from build123d import *

# Parameters (mm, degrees)
F0_R     = 13.57391
F1_DEPTH = 17
F3_DEPTH = 1.5
F5_DEPTH = 34
F6_R     = 1
F7_R     = 15.57391
F7_R_2   = 13.57391
F8_DEPTH = 1.5
F9_SIZE2 = 0.99999
F9_SIZE  = 1.99999
F10_R    = 1


# Not quite as in the source:
# - a fillet or chamfer is up to 0.001 mm smaller than in the source, because OpenCascade refuses the exact size
# - a feature names something its author has since deleted; it is built from what else it names


with BuildPart() as f1:
    # F0 (on Top) → F1 (new body, symmetric)
    with BuildSketch(Plane.XY):
        Circle(F0_R)
    extrude(amount=F1_DEPTH, both=True)

    # F2 (on Top) → F3 (join, symmetric)
    with BuildSketch(Plane.XY):
        with BuildLine():
            Line((-8.8722387473, 10.27299432), (-13.094084175, 11.721231689))
            ThreePointArc((-13.094084175, 11.721231689), (-13.7398361081, 10.9571536638), (-14.3410637787, 10.1575687241))
            Line((-14.3410637787, 10.1575687241), (-11.9896877566, 6.3638369077))
            ThreePointArc((-11.9896877566, 6.3638369077), (-10.6125101782, 8.4631944563), (-8.8722387473, 10.27299432))
        make_face()
        with BuildLine():
            ThreePointArc((1, 17.5454356654), (0, 17.57391), (-1, 17.5454356654))
            Line((-1, 17.5454356654), (-2.5, 13.3417027657))
            ThreePointArc((-2.5, 13.3417027657), (0, 13.57391), (2.5, 13.3417027657))
            Line((2.5, 13.3417027657), (1, 17.5454356654))
        make_face()
        with BuildLine():
            Line((11.9896877566, 6.3638369077), (14.3410637787, 10.1575687241))
            ThreePointArc((14.3410637787, 10.1575687241), (13.7398361081, 10.9571536638), (13.094084175, 11.721231689))
            Line((13.094084175, 11.721231689), (8.8722387473, 10.27299432))
            ThreePointArc((8.8722387473, 10.27299432), (10.6125101782, 8.4631944563), (11.9896877566, 6.3638369077))
        make_face()
        with BuildLine():
            Line((12.4508960874, -5.4061279404), (16.8830140276, -4.8791546431))
            ThreePointArc((16.8830140276, -4.8791546431), (17.1332953852, -3.9105628665), (17.3280558955, -2.9292988187))
            Line((17.3280558955, -2.9292988187), (13.5635007572, -0.5314883795))
            ThreePointArc((13.5635007572, -0.5314883795), (13.2335837364, -3.0204791306), (12.4508960874, -5.4061279404))
        make_face()
        with BuildLine():
            Line((3.5363257124, -13.1051681845), (6.711710363, -16.2417750474))
            ThreePointArc((6.711710363, -16.2417750474), (7.6250337817, -15.8335457973), (8.5136480988, -15.3740075692))
            Line((8.5136480988, -15.3740075692), (8.0411700519, -10.9357494889))
            ThreePointArc((8.0411700519, -10.9357494889), (5.8894988252, -12.2296703257), (3.5363257124, -13.1051681845))
        make_face()
        with BuildLine():
            Line((-8.0411700519, -10.9357494889), (-8.5136480988, -15.3740075692))
            ThreePointArc((-8.5136480988, -15.3740075692), (-7.6250337817, -15.8335457973), (-6.711710363, -16.2417750474))
            Line((-6.711710363, -16.2417750474), (-3.5363257124, -13.1051681845))
            ThreePointArc((-3.5363257124, -13.1051681845), (-5.8894988252, -12.2296703257), (-8.0411700519, -10.9357494889))
        make_face()
        with BuildLine():
            Line((-13.5635007572, -0.5314883795), (-17.3280558955, -2.9292988187))
            ThreePointArc((-17.3280558955, -2.9292988187), (-17.1332953852, -3.9105628665), (-16.8830140276, -4.8791546431))
            Line((-16.8830140276, -4.8791546431), (-12.4508960874, -5.4061279404))
            ThreePointArc((-12.4508960874, -5.4061279404), (-13.2335837364, -3.0204791306), (-13.5635007572, -0.5314883795))
        make_face()
    extrude(amount=F3_DEPTH, both=True)

    # F4 (on face) → F5 (cut)
    with BuildSketch(Plane.XY.offset(17)):
        with BuildLine():
            ThreePointArc((-3.0007085232, 1.5847516846), (-2.6531275445, 2.1157986141), (-2.2127391143, 2.5728340707))
            Line((-2.2127391143, 2.5728340707), (-6.6382173429, 7.718502212))
            ThreePointArc((-6.6382173429, 7.718502212), (-7.9593826336, 6.3473958423), (-9.0021255696, 4.7542550537))
            Line((-9.0021255696, 4.7542550537), (-3.0007085232, 1.5847516846))
        make_face()
        with BuildLine():
            ThreePointArc((-0.6319024037, 3.334124907), (-0.3173418417, 3.3786067688), (0, 3.3934775))
            Line((0, 3.3934775), (0, 6.786955))
            Line((0, 6.786955), (0, 10.1804325))
            ThreePointArc((0, 10.1804325), (-0.9520255252, 10.1358203065), (-1.895707211, 10.0023747209))
            Line((-1.895707211, 10.0023747209), (-0.6319024037, 3.334124907))
        make_face()
        with BuildLine():
            Line((0, 6.786955), (0, 3.3934775))
            ThreePointArc((0, 3.3934775), (0.3173418417, 3.3786067688), (0.6319024037, 3.334124907))
            Line((0.6319024037, 3.334124907), (1.895707211, 10.0023747209))
            ThreePointArc((1.895707211, 10.0023747209), (0.9520255252, 10.1358203065), (0, 10.1804325))
            Line((0, 10.1804325), (0, 6.786955))
        make_face()
        with BuildLine():
            ThreePointArc((2.2127391143, 2.5728340707), (2.6531275445, 2.1157986141), (3.0007085232, 1.5847516846))
            Line((3.0007085232, 1.5847516846), (9.0021255696, 4.7542550537))
            ThreePointArc((9.0021255696, 4.7542550537), (7.9593826336, 6.3473958423), (6.6382173429, 7.718502212))
            Line((6.6382173429, 7.718502212), (2.2127391143, 2.5728340707))
        make_face()
        with BuildLine():
            ThreePointArc((3.3911429475, -0.1258532971), (3.3083959341, -0.7551197827), (3.1099199215, -1.3579718793))
            Line((3.1099199215, -1.3579718793), (9.3297597644, -4.073915638))
            ThreePointArc((9.3297597644, -4.073915638), (9.9251878023, -2.265359348), (10.1734288426, -0.3775598913))
            Line((10.1734288426, -0.3775598913), (3.3911429475, -0.1258532971))
        make_face()
        with BuildLine():
            ThreePointArc((2.0159469746, -2.7297705652), (1.4723747063, -3.0574175814), (0.8772981881, -3.2781149205))
            Line((0.8772981881, -3.2781149205), (2.6318945642, -9.8343447616))
            ThreePointArc((2.6318945642, -9.8343447616), (4.4171241189, -9.1722527443), (6.0478409237, -8.1893116956))
            Line((6.0478409237, -8.1893116956), (2.0159469746, -2.7297705652))
        make_face()
        with BuildLine():
            ThreePointArc((-0.8772981881, -3.2781149205), (-1.4723747063, -3.0574175814), (-2.0159469746, -2.7297705652))
            Line((-2.0159469746, -2.7297705652), (-6.0478409237, -8.1893116956))
            ThreePointArc((-6.0478409237, -8.1893116956), (-4.4171241189, -9.1722527443), (-2.6318945642, -9.8343447616))
            Line((-2.6318945642, -9.8343447616), (-0.8772981881, -3.2781149205))
        make_face()
        with BuildLine():
            ThreePointArc((-3.1099199215, -1.3579718793), (-3.3083959341, -0.7551197827), (-3.3911429475, -0.1258532971))
            Line((-3.3911429475, -0.1258532971), (-10.1734288426, -0.3775598913))
            ThreePointArc((-10.1734288426, -0.3775598913), (-9.9251878023, -2.265359348), (-9.3297597644, -4.073915638))
            Line((-9.3297597644, -4.073915638), (-3.1099199215, -1.3579718793))
        make_face()
        Polygon((1.3273298856, 0.7009971998), (0, 0), (1.6957169725, -0.0629320484), (1.7320508076, 0), align=None)
        Polygon((1.6957169725, -0.0629320484), (0, 0), (1.3833114811, -0.6040342321), align=None)
        Polygon((1.3833114811, -0.6040342321), (0, 0), (0.9720883359, -1.3162936127), align=None)
        Polygon((0.9720883359, -1.3162936127), (0, 0), (0.4014341516, -1.5), (0.8660254038, -1.5), align=None)
        Polygon((0.4014341516, -1.5), (0, 0), (-0.4014341516, -1.5), align=None)
        Polygon((-0.4014341516, -1.5), (0, 0), (-0.9720883359, -1.3162936127), (-0.8660254038, -1.5), align=None)
        Polygon((-0.9720883359, -1.3162936127), (0, 0), (-1.3833114811, -0.6040342321), align=None)
        Polygon((-1.3833114811, -0.6040342321), (0, 0), (-1.6957169725, -0.0629320484), align=None)
        Polygon((-1.6957169725, -0.0629320484), (0, 0), (-1.3273298856, 0.7009971998), (-1.7320508076, 0), align=None)
        Polygon((-1.3273298856, 0.7009971998), (0, 0), (-1.0363453205, 1.2049972508), align=None)
        Polygon((-1.0363453205, 1.2049972508), (0, 0), (-0.2842885711, 1.5), (-0.8660254038, 1.5), align=None)
        Polygon((-0.2842885711, 1.5), (0, 0), (0, 1.5), align=None)
        Polygon((0, 1.5), (0, 0), (0.2842885711, 1.5), align=None)
        Polygon((0.2842885711, 1.5), (0, 0), (1.0363453205, 1.2049972508), (0.8660254038, 1.5), align=None)
        Polygon((1.0363453205, 1.2049972508), (0, 0), (1.3273298856, 0.7009971998), align=None)
    extrude(amount=-F5_DEPTH, mode=Mode.SUBTRACT)

    # F6
    f6_edges = [f1.edges().sort_by_distance(p)[0] for p in [
        (-6.047841, -8.189312, 0),
        (-2.631895, -9.834345, 0),
        (2.631895, -9.834345, 0),
        (6.047841, -8.189312, 0),
        (9.32976, -4.073916, 0),
        (-9.32976, -4.073916, 0),
        (-10.173429, -0.37756, 0),
        (-9.002126, 4.754255, 0),
        (-6.638217, 7.718502, 0),
        (6.638217, 7.718502, 0),
        (-1.895707, 10.002375, 0),
        (1.895707, 10.002375, 0),
        (9.002126, 4.754255, 0),
        (10.173429, -0.37756, 0),
    ]]
    fillet(f6_edges, radius=F6_R)

    # F7 (on face) → F8 (join)
    with BuildSketch(Plane(origin=(0, 0, -17), x_dir=(1, 0, 0), z_dir=(0, 0, -1))):
        Circle(F7_R)
        Circle(F7_R_2, mode=Mode.SUBTRACT)
    extrude(amount=-F8_DEPTH)

    # F9 (size 2 and 1 in the source; OpenCascade refuses exactly that, so slightly less here)
    f9_edges = [f1.edges().sort_by_distance(p)[0] for p in [
        (-15.57391, 0, -15.5),
    ]]
    f9_side = f1.faces().sort_by_distance((-15.133413, 0, -15.5))[0]
    chamfer(f9_edges, length=F9_SIZE, length2=F9_SIZE2, reference=f9_side)

    # F10
    f10_edges = [f1.edges().sort_by_distance(p)[0] for p in [
        (14.341064, 10.157569, 0),
        (13.094084, 11.721232, 0),
        (1, 17.545436, 0),
        (-1, 17.545436, 0),
        (-13.094084, 11.721232, 0),
        (-14.341064, 10.157569, 0),
        (-17.328056, -2.929299, 0),
        (-16.883014, -4.879155, 0),
        (-8.513648, -15.374008, 0),
        (-6.71171, -16.241775, 0),
        (6.71171, -16.241775, 0),
        (8.513648, -15.374008, 0),
        (16.883014, -4.879155, 0),
        (17.328056, -2.929299, 0),
    ]]
    fillet(f10_edges, radius=F10_R)


solid = f1.part
CAD build for the part. Positions are in the model's coordinates, mm. A direction names the side the tool comes from. Give positions to 0.01 mm unless a question says otherwise; leave off trailing zeros. Return JSON: item names as keys, results as strings.
Item 1: Drill centre lines: probe 1 along Y at (x, z) = (7.5, -11.5); probe 2 along Y at (x, z) = (-5, 8); probe 3 along X at (y, z) = (-0.5, -15). Where is each one in solid material? Low to high.
Answer below:
{"probe 1": "y = -11.31 to -3.27, -0.28 to 3.96, 6.88 to 11.31", "probe 2": "y = -12.62 to -8.87, -6.77 to -2.18, -0.19 to 2.64, 5.81 to 12.62", "probe 3": "x = -13.56 to -9.63, -3.36 to -1.44, 1.44 to 3.36, 9.63 to 13.56"}
Item 2: Two-plate mould, pull along X, no slides. Class faces 1 (the cylindrical face through (8.33, -15.28, 0.02)), 2 (the flat face through (-14.36, -5.18, 0.02)), 3 (the flat face through (4.11, 4.78, 0.24)), 4 (the flat face through (-15, -3, -1.5)): +X half, -X half, draft (parallel to the pull), parting line (faces both ways), or undercut.
Answer below:
{"face 1": "+X half", "face 2": "-X half", "face 3": "undercut", "face 4": "draft"}
Item 3: Drop flat-ended pins along their axis: pin 1 (1.6 mm diameter, centred on x = -12.5, y = 9.5, fed in from +Z); pin 2 (5 mm diameter, centred on x = -5.5, z = -6.5, fed in from +Y); pin 3 (4 mm diameter, centred on x = -7, z = 13.5, fed in from +Y). Give the stop position or say it passes through.
Answer below:
{"pin 1": "stops at z = 1.5", "pin 2": "stops at y = 13.24", "pin 3": "stops at y = 12.62"}
Item 4: Band-saw the part on A-A (z = 5). Give the number of separate pieces and of enclosed holes in the cut face, then the cut area to 3 significant figures.
Answer below:
{"separate pieces": "1", "enclosed holes": "8", "area": "454 mm2"}
Item 5: Tool access for faces 5 (the flat face through (-15, -3, 1.5)), 6 (the flat face through (-13.001, 7.995, -0.021)), 7 (the flat face through (6.295, -0.234, 0.238)), 8 (the flat face through (0, -3, 17)), 9 (the flat face through (-7, -14, -1.5)): list every direction of +Z, -Z, +X, -X, +Y, -Y with a clear straight run to the whole face (end or side of a thin tool).
Answer below:
{"face 5": "+Z, -X, -Y", "face 6": "+Z, -X", "face 7": "+Z, -Z", "face 8": "+Z, +X, -X, +Y, -Y", "face 9": "-X, -Y"}
